Read the model definition and answer for the solid it produces. Units are mm, in the model's axes. A direction names the side the tool comes from. Give positions to 0.01 mm unless a question says otherwise; leave off trailing zeros. Order: outer loops, then holes, each group sorted by start corner. A loop starts at its lowest first (then second) coordinate and runs counter-clockwise, first axis right, second up. Notation, with made-up numbers: (-18, -1.75) - (21, -1.75) arc R17 ccw to (21, 20.25) - close; hole circle Ø6 at (-17, 48). An arc over 180 degrees is marked (long way). Write each question's results on one line, items separated by ' | '.
from build123d import *

# Parameters (mm, degrees)
SKETCH1_R           = 11.176
BASE_EXTRUDE_DEPTH  = 6.35
SHELL1_T            = 1.778
FILLET1_R           = 0.889
BOSS_EXTRUDE1_REACH = 41.555
SKETCH2_R           = 6.35
CUT_EXTRUDE1_DEPTH  = 10.795
BOSS_EXTRUDE2_REACH = 37.383
SKETCH4_R           = 4.445
SKETCH5_R           = 3.175
CUT_EXTRUDE2_DEPTH  = 2.159
CUT_EXTRUDE3_REACH  = 31.183
SKETCH6_R           = 1.5875


with BuildPart() as part:
    # Sketch1 → Base-Extrude (new, symmetric)
    with BuildSketch(Plane.XY):
        Circle(SKETCH1_R)
    extrude(amount=BASE_EXTRUDE_DEPTH, both=True)

    # Shell1
    shell1_openings = [part.faces().sort_by_distance(p)[0] for p in [
        (0, 0, 6.35),
        (0, 0, -6.35),
    ]]
    offset(amount=SHELL1_T, openings=shell1_openings, kind=Kind.INTERSECTION)

    # Fillet1
    # the kernel refuses this fillet: 0.889 mm, written as the material it takes off along each edge
    with BuildSketch(Plane(origin=(0, 0, -6.35), x_dir=(1, 0, 0), z_dir=(0, -1, 0))) as fillet1_piece_1:
        with BuildLine():
            CenterArc((12.954 - FILLET1_R, FILLET1_R), FILLET1_R, 270, 90)
            Line((12.954 - FILLET1_R, 0), (12.954, 0))
            Line((12.954, 0), (12.954, FILLET1_R))
        make_face()
    revolve(axis=Axis((0, 0, -6.35), (0, 0, 1)), mode=Mode.SUBTRACT)
    with BuildSketch(Plane(origin=(0, 0, 6.35), x_dir=(1, 0, 0), z_dir=(0, -1, 0))) as fillet1_piece_2:
        with BuildLine():
            CenterArc((12.954 - FILLET1_R, -FILLET1_R), FILLET1_R, 0, 90)
            Line((12.954, -FILLET1_R), (12.954, 0))
            Line((12.954, 0), (12.954 - FILLET1_R, 0))
        make_face()
    revolve(axis=Axis((0, 0, 6.35), (0, 0, 1)), mode=Mode.SUBTRACT)
    with BuildSketch(Plane(origin=(0, 0, -6.35), x_dir=(1, 0, 0), z_dir=(0, -1, 0))) as fillet1_piece_3:
        with BuildLine():
            CenterArc((11.176 + FILLET1_R, FILLET1_R), FILLET1_R, 180, 90)
            Line((11.176 + FILLET1_R, 0), (11.176, 0))
            Line((11.176, 0), (11.176, FILLET1_R))
        make_face()
    revolve(axis=Axis((0, 0, -6.35), (0, 0, 1)), mode=Mode.SUBTRACT)
    with BuildSketch(Plane(origin=(0, 0, 6.35), x_dir=(1, 0, 0), z_dir=(0, -1, 0))) as fillet1_piece_4:
        with BuildLine():
            CenterArc((11.176 + FILLET1_R, -FILLET1_R), FILLET1_R, 90, 90)
            Line((11.176 + FILLET1_R, 0), (11.176, 0))
            Line((11.176, 0), (11.176, -FILLET1_R))
        make_face()
    revolve(axis=Axis((0, 0, 6.35), (0, 0, 1)), mode=Mode.SUBTRACT)

    # Sketch2 → Boss-Extrude1 (add, up to next)
    with BuildSketch(Plane(origin=(0, -23.876, 0), x_dir=(-1, 0, 0), z_dir=(0, 1, 0)), mode=Mode.PRIVATE) as boss_extrude1_sk1:
        with Locations(Location((0, 0, 0), (0, 0, 90))):
            Circle(SKETCH2_R)
    boss_extrude1_tool1 = extrude(boss_extrude1_sk1.sketch, amount=BOSS_EXTRUDE1_REACH, mode=Mode.PRIVATE) - part.part
    add(boss_extrude1_tool1.solids().sort_by_distance((0, -23.876, 0))[0])

    # Sketch3 → Cut-Extrude1 (cut)
    with BuildSketch(Plane.XZ.offset(23.876)):
        with BuildLine():
            Line((-1.5875, 3.60275072), (1.5875, 3.60275072))
            ThreePointArc((1.5875, 3.60275072), (0, -3.937), (-1.5875, 3.60275072))
        make_face()
    extrude(amount=-CUT_EXTRUDE1_DEPTH, mode=Mode.SUBTRACT)

    # Sketch4 → Boss-Extrude2 (add, up to next)
    with BuildSketch(Plane(origin=(0, -17.371432399, 6.477), x_dir=(-1, 0, 0), z_dir=(0, 0, 1)), mode=Mode.PRIVATE) as boss_extrude2_sk1:
        with Locations(Location((0, 0.789567601, 0), (0, 0, 180))):
            Circle(SKETCH4_R)
    boss_extrude2_tool1 = extrude(boss_extrude2_sk1.sketch, amount=-BOSS_EXTRUDE2_REACH, mode=Mode.PRIVATE) - part.part
    add(boss_extrude2_tool1.solids().sort_by_distance((0, -18.161, 6.477))[0])

    # Sketch5 → Cut-Extrude2 (cut)
    with BuildSketch(Plane.XY.offset(6.477)):
        with Locations((0, -18.161)):
            Circle(SKETCH5_R)
    extrude(amount=-CUT_EXTRUDE2_DEPTH, mode=Mode.SUBTRACT)

    # Sketch6 → Cut-Extrude3 (cut, up to next)
    with BuildSketch(Plane.XY.offset(4.318), mode=Mode.PRIVATE) as cut_extrude3_sk1:
        with Locations((0, -18.161)):
            Circle(SKETCH6_R)
    cut_extrude3_tool1 = extrude(cut_extrude3_sk1.sketch, amount=-CUT_EXTRUDE3_REACH, mode=Mode.PRIVATE) & part.part
    add(cut_extrude3_tool1.solids().sort_by_distance((0, -18.161, 4.318))[0], mode=Mode.SUBTRACT)


solid = part.part
(1) The mould has two halves that part along Z. Classify faces 4 (the face through (0, -22, 3.603)), 5 (the face through (0.279, -17.672, -6.344)), 6 (the face through (-8.87, -6.8, 0.08)): pulls with the +Z half, pulls with the -Z half, needs draft (parallel to the pull), parting line crosses it, or undercut.
Conclusion:
face 4: undercut | face 5: parting line crosses it | face 6: needs draft
(2) Section B-B (z = 0) is taken. Give the vertices of the cut face in (x, y).
Conclusion:
outline: (-6.35, -23.88) - (-3.94, -23.88) - (-3.94, -13.08) - (3.94, -13.08) - (3.94, -23.88) - (6.35, -23.88) - (6.35, -11.29) arc R12.95 ccw (long way) to (-6.35, -11.29) - close; hole circle Ø22.35 at (0, 0)
(3) Section C-C (x = 0) is taken. State how many separate pieces and enclosed holes the cut face has, plus the area to 3 significant figures.
Conclusion:
separate pieces: 3 | enclosed holes: 0 | area: 86.6 mm^2
(4) For faces 1 (the face through (-0.69, -21.26, 5.41)), 2 (the face through (0.15, -18.554, -3.934)), 3 (the face through (3, -20, 6.477)), determine the directions among +Z, -Z, +X, -X, +Y, -Y from which every point of the face is accessible in a straight line to the end or side of a thin tool.
Conclusion:
face 1: +Z | face 2: -Y | face 3: +Z, +X, -X, +Y, -Y
(5) Each of these flat-tipped pins is pushed along its axis until it touches: pin 1 (2 mm diameter, centred on x = -0.5, z = 1, fed in from -Y); pin 2 (5 mm diameter, centred on x = 0, y = -18.161, fed in from +Z); pin 3 (4 mm diameter, centred on x = -2.5, z = -5, fed in from +Y); pin 4 (4 mm diameter, centred on x = 9.5, y = -16, fed in from +Z). Where does it stop, or does it pass through?
Conclusion:
pin 1: y = -13.08 | pin 2: z = 4.32 | pin 3: y = 12.94 | pin 4: through
(6) Consider probe 1 along Y at (x, z) = (0, 3.9); probe 2 along X at (y, z) = (-19.5, -0.25); probe 3 along Y at (x, z) = (-1.5, 5). Determine where each line is inside the solid, lowest interval first. Write a range as [from, to].
Conclusion:
probe 1: [-23.88, -19.75], [-16.57, -11.18], [11.18, 12.95] | probe 2: [-6.35, -3.93], [3.93, 6.35] | probe 3: [-23.88, -20.96], [-15.36, -11.07], [11.07, 12.87]
(7) Section D-D (z = 2.5) is taken. Give the vertices of the cut face in (x, y).
Conclusion:
outline: (-5.84, -23.88) - (-3.04, -23.88) - (-3.04, -13.08) - (3.04, -13.08) - (3.04, -23.88) - (5.84, -23.88) - (5.84, -11.56) arc R12.95 ccw (long way) to (-5.84, -11.56) - close; hole circle Ø22.35 at (0, 0)
(8) Section A-A (y = 0) is taken. Give the vertices of the cut face in (x, z) (3 decimals).
Conclusion:
outline: (-12.954, -5.461) arc R0.889 ccw to (-11.176, -5.461) - (-11.176, 5.461) arc R0.889 ccw to (-12.954, 5.461) - close; (11.176, -5.461) arc R0.889 ccw to (12.954, -5.461) - (12.954, 5.461) arc R0.889 ccw to (11.176, 5.461) - close
